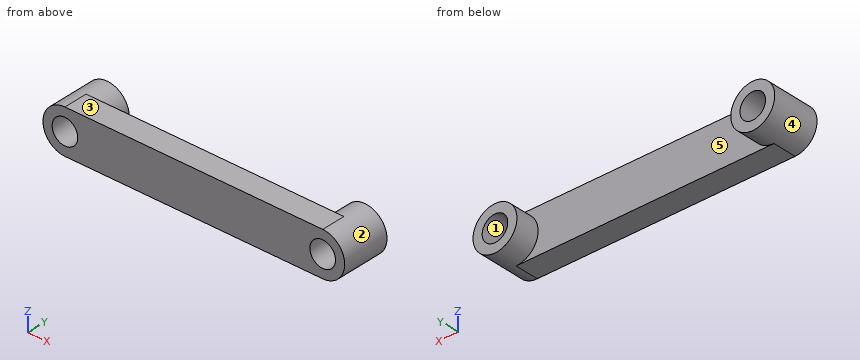
from build123d import *

# Parameters (mm, degrees)
CROQUIS1_R              = 1.6
SALIENTE_EXTRUIR1_DEPTH = 3
CROQUIS2_R              = 2.75
CROQUIS2_R_2            = 1.6
SALIENTE_EXTRUIR2_DEPTH = 3


with BuildPart() as part:
    # Croquis1 → Saliente-Extruir1 (new body)
    with BuildSketch(Plane(origin=(0, 0, 0), x_dir=(1, 0, 0), z_dir=(0, 1, 0))):
        with BuildLine():
            ThreePointArc((0, 2.75), (-2.75, 0), (0, -2.75))
            Line((0, -2.75), (32.26, -2.75))
            ThreePointArc((32.26, -2.75), (35.01, 0), (32.26, 2.75))
            Line((32.26, 2.75), (0, 2.75))
        make_face()
        with Locations(Location((0, 0, 0), (0, 0, 270))):
            Circle(CROQUIS1_R, mode=Mode.SUBTRACT)
        with Locations(Location((32.26, 0, 0), (0, 0, 270))):
            Circle(CROQUIS1_R, mode=Mode.SUBTRACT)
    extrude(amount=SALIENTE_EXTRUIR1_DEPTH)

    # Croquis2 → Saliente-Extruir2 (add)
    # profile 1 of 2: a face of its own
    with BuildSketch(Plane(origin=(0, 3, 0), x_dir=(1, 0, 0), z_dir=(0, 1, 0))):
        with Locations(Location((0, 0, 0), (0, 0, 270))):
            Circle(CROQUIS2_R)
        with Locations(Location((0, 0, 0), (0, 0, 270))):
            Circle(CROQUIS2_R_2, mode=Mode.SUBTRACT)
    # profile 2 of 2: a face of its own
    with BuildSketch(Plane(origin=(0, 3, 0), x_dir=(1, 0, 0), z_dir=(0, 1, 0))):
        with Locations(Location((32.26, 0, 0), (0, 0, 270))):
            Circle(CROQUIS2_R)
        with Locations(Location((32.26, 0, 0), (0, 0, 270))):
            Circle(CROQUIS2_R_2, mode=Mode.SUBTRACT)
    extrude(amount=SALIENTE_EXTRUIR2_DEPTH)


solid = part.part
Read the model definition and answer for the solid it produces. Units are mm, in the model's axes. Face numbers are marked on the shaded views. A direction names the side the tool comes from. Give positions to 0.01 mm unless a question says otherwise; leave off trailing zeros. Loops run counter-clockwise (first coordinate to the right, second up) from the corner with the lowest first, then second, coordinate; pieces in that order, holes last. Notation, with made-up numbers: (41, 80.25) -> (56, 80.25) arc R10 cw to (56, 87.25) -> close; hole circle Ø1 at (8, -8.75). An arc over 180 degrees is marked (long way). Use a Markdown table: item, result.
Q1. Section B-B, the plane y = 4.1 is taken. Determine the outline of the cut face in (x, z), then the cut area to 3 significant figures.
Solved:
| item | result |
|---|---|
| outline | circle Ø5.5 at (0, 0); circle Ø5.5 at (32.26, 0); hole circle Ø3.2 at (0, 0); hole circle Ø3.2 at (32.26, 0) |
| area | 31.4 mm^2 |
Q2. Section D-D, the plane x = 14 is taken. Determine the outline of the cut face in (y, z).
Solved:
| item | result |
|---|---|
| outline | (0, -2.75) -> (3, -2.75) -> (3, 2.75) -> (0, 2.75) -> close |
Q3. Determine the mould class of the marked faces 3, 4 and 5 for opening direction X: pulls with the +X half, pulls with the -X half, needs draft (parallel to the pull), parting line crosses it, or undercut.
Solved:
| item | result |
|---|---|
| face 3 | needs draft |
| face 4 | undercut |
| face 5 | undercut |
Q4. A tool of negligible diameter and unlimited length cuts with its end or side. For the marked faces 1 and 2, from which of +Z, -Z, +X, -X, +Y, -Y can it reach the whole face along a straight path? Write none if from no direction.
Solved:
| item | result |
|---|---|
| face 1 | +Y, -Y |
| face 2 | +Y |
Q5. Section C-C, the plane y = 1.7 is taken. Determine the outline of the cut face in (x, z), then the cut area to 3 significant figures.
Solved:
| item | result |
|---|---|
| outline | (0, -2.75) -> (32.26, -2.75) arc R2.75 ccw to (32.26, 2.75) -> (0, 2.75) arc R2.75 ccw to start; hole circle Ø3.2 at (0, 0); hole circle Ø3.2 at (32.26, 0) |
| area | 185 mm^2 |
Q6. Find the intervals of material crossed by line 1 along X through (y, z) = (1.2, 0); line 2 along X through (y, z) = (4.15, 0); line 3 along Y through (x, z) = (6.5, -2.3), in increasing order.
Solved:
| item | result |
|---|---|
| line 1 | x = -2.75 to -1.6, 1.6 to 30.66, 33.86 to 35.01 |
| line 2 | x = -2.75 to -1.6, 1.6 to 2.75, 29.51 to 30.66, 33.86 to 35.01 |
| line 3 | y = 0 to 3 |
